Could you check a few things on this drawing? It's one solid part, dimensions in mm from its lowest x, y, z. Round coordinates to 2 decimals unless told otherwise and drop trailing zeros. Loops run counter-clockwise (first coordinate to the right, second up) from the corner with the lowest first, then second, coordinate; pieces in that order, holes last. Notation, with made-up numbers: M 50.25,-11 L 104.25,-11 A18 ccw 104.25,4 Z; hole C -31.5,-32.75 d1. An arc over 180 degrees is marked long. Answer as a JSON object with one key per item and string values.
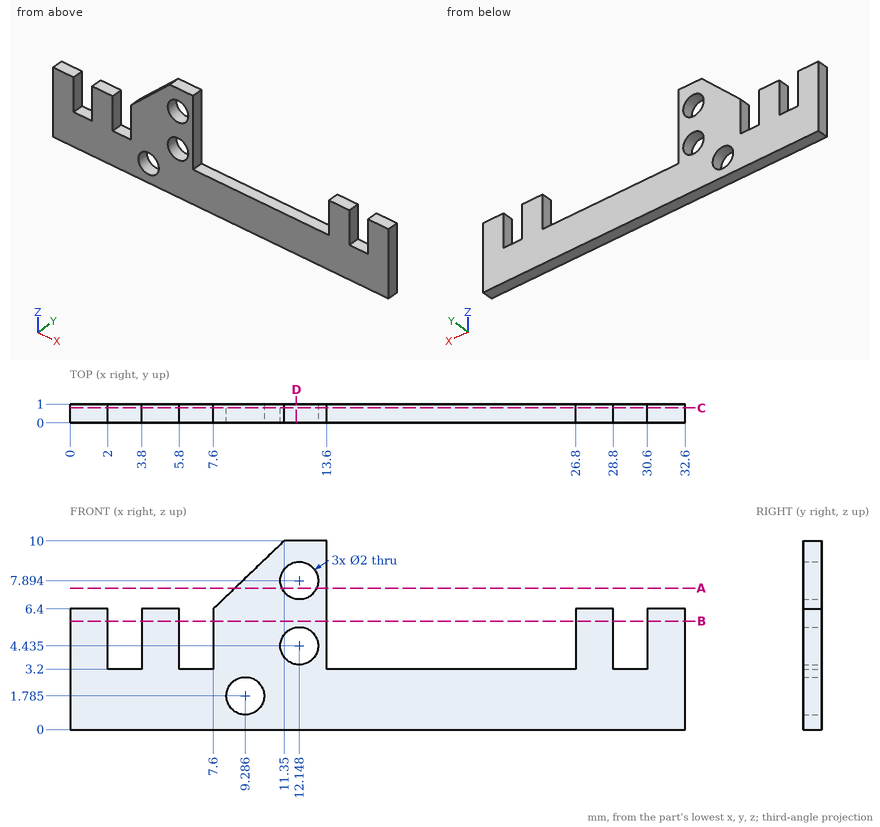
Item 1: I'm going to push flat-ended pins straight in: pin 1 Ø0.5 at (x, y) = (7, 0.5) entering from +Z; pin 2 Ø3 at (x, z) = (21.5, 4) entering from +Y. Where does each tip first touch, or does it pass through?
Resolved:
{"pin 1": "z = 3.2", "pin 2": "y = 1"}
Item 2: I want a section at D-D, the plane x = 12. Please give me the cut outline in (y, z) (1 decimal).
Resolved:
{"outline": "M 0,0 L 1,0 L 1,3.4 L 0,3.4 Z; M 0,5.4 L 1,5.4 L 1,6.9 L 0,6.9 Z; M 0,8.9 L 1,8.9 L 1,10 L 0,10 Z"}
Item 3: I want a section at A-A, the plane z = 7.5. Please give me the cut outline in (x, y) (1 decimal).
Resolved:
{"outline": "M 8.7,0 L 11.2,0 L 11.2,1 L 8.7,1 Z; M 13.1,0 L 13.6,0 L 13.6,1 L 13.1,1 Z"}
Item 4: I want a section at B-B, the plane z = 5.75. Please give me the cut outline in (x, y), then the cut area to 3 significant figures.
Resolved:
{"outline": "M 0,0 L 2,0 L 2,1 L 0,1 Z; M 3.8,0 L 5.8,0 L 5.8,1 L 3.8,1 Z; M 7.6,0 L 13.6,0 L 13.6,1 L 7.6,1 Z; M 26.8,0 L 28.8,0 L 28.8,1 L 26.8,1 Z; M 30.6,0 L 32.6,0 L 32.6,1 L 30.6,1 Z", "area": "14.0 mm²"}
Item 5: Please list where these lines run through material, in increasing order: probe 1 along X at (y, z) = (0.1, 5.75); probe 2 along X at (y, z) = (0.1, 5.25) (1 decimal); probe 3 along Z at (x, y) = (12, 0.7) (1 decimal). Write a range as from..to.
Resolved:
{"probe 1": "0..2, 3.8..5.8, 7.6..13.6, 26.8..28.8, 30.6..32.6", "probe 2": "0..2, 3.8..5.8, 7.6..11.6, 12.7..13.6, 26.8..28.8, 30.6..32.6", "probe 3": "0..3.4, 5.4..6.9, 8.9..10"}
Item 6: I want a section at C-C, the plane y = 0.8. State how many separate pieces and enclosed holes the cut face has.
Resolved:
{"separate pieces": "1", "enclosed holes": "3"}
